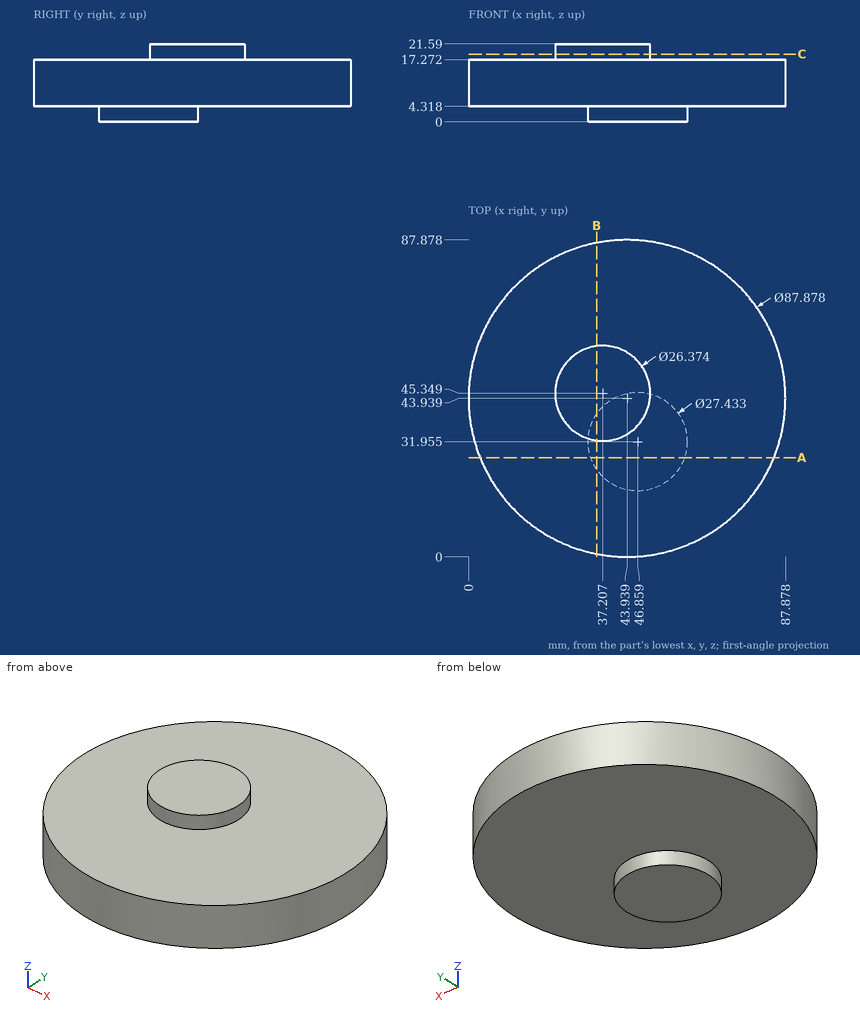
Geometry: see drawing. Coordinates: mm, zero at the bounding-box minimum. Coordinates: 2 decimals unless noted, no trailing zeros. Order: outer loops, then holes, each group sorted by start corner. A loop starts at its lowest first (then second) coordinate and runs counter-clockwise, first axis right, second up. Notation, with made-up numbers: M 86.5,0 L 106.5,0 A17 cw 106.5,4 Z; hole C 13.25,69.25 d10. An arc over 180 degrees is marked long. Write each question's results on one line, items separated by ' | '. Start each with the question number.
1) Section query B-B (x = 35.5). Return the cut outline in (y, z) (1 decimal), plus the area to 3 significant figures.
2) Section query A-A (y = 27.5). Return the cut outline in (x, z).
3) Line query: line 1 (Z direction, x = 39.5, y = 17); line 2 (Y direction, x = 44.5, z = 8) (1 decimal); line 3 (X direction, y = 6.5, z = 10) (1 decimal). Output: solid intervals per line, ascending. Write a range as from..to.
4) Section query C-C (z = 18.75). Return the cut outline in (x, y).
5) Contact query for flat-ended pins moving along their axis: pin 1 Ø6 at (y, z) = (38.5, 16.5) entering from +X; pin 2 Ø6 at (y, z) = (28.5, 6) entering from +X; pin 3 Ø4 at (y, z) = (38, 14) entering from -X. Output: stop coordinate, or through.
Answers:
1) outline: M 0.8,4.3 L 24.3,4.3 L 24.3,0 L 39.6,0 L 39.6,4.3 L 87.1,4.3 L 87.1,17.3 L 58.4,17.3 L 58.4,21.6 L 32.3,21.6 L 32.3,17.3 L 0.8,17.3 Z | area: 1,300 mm^2
2) outline: M 3.19,4.32 L 33.89,4.32 L 33.89,0 L 59.83,0 L 59.83,4.32 L 84.69,4.32 L 84.69,17.27 L 3.19,17.27 Z
3) line 1: z = 4.32..17.27 | line 2: y = 0..87.9 | line 3: x = 20.9..66.9
4) outline: C 37.21,45.35 d26.37
5) pin 1: stops at x = 87.81 | pin 2: stops at x = 86.08 | pin 3: stops at x = 0.18
